from build123d import *

# Parameters (mm, degrees)
SKETCH1_W           = 96
SKETCH1_H           = 48
SKETCH1_R           = 2.05
BOSS_EXTRUDE1_DEPTH = 3.175
FILLET1_R           = 2


with BuildPart() as part:
    # Sketch1 → Boss-Extrude1 (new body)
    with BuildSketch(Plane.XY):
        Rectangle(SKETCH1_W, SKETCH1_H)
        with Locations((-40, 16)):
            Circle(SKETCH1_R, mode=Mode.SUBTRACT)
        with Locations((-8, 16)):
            Circle(SKETCH1_R, mode=Mode.SUBTRACT)
        with Locations((-8, -16)):
            Circle(SKETCH1_R, mode=Mode.SUBTRACT)
        with Locations((-40, -16)):
            Circle(SKETCH1_R, mode=Mode.SUBTRACT)
        with Locations((8, 16)):
            Circle(SKETCH1_R, mode=Mode.SUBTRACT)
        with Locations((8, -16)):
            Circle(SKETCH1_R, mode=Mode.SUBTRACT)
        with Locations((40, -16)):
            Circle(SKETCH1_R, mode=Mode.SUBTRACT)
        with Locations((40, 16)):
            Circle(SKETCH1_R, mode=Mode.SUBTRACT)
        with Locations((-36.7, 0)):
            Circle(SKETCH1_R, mode=Mode.SUBTRACT)
        with Locations((11.3, 0)):
            Circle(SKETCH1_R, mode=Mode.SUBTRACT)
        Polygon((-38.544929421, 20.05), (-30, 13), (-30, -13), (-38.544929421, -20.05), (-9.455070579, -20.05), (-18, -13), (-18, 13), (-9.455070579, 20.05), align=None, mode=Mode.SUBTRACT)
        Polygon((-11, -6), (-11, 6), (-4, 14.484327085), (4, 14.484327085), (4, -14.484327085), (-4, -14.484327085), align=None, mode=Mode.SUBTRACT)
        Polygon((38.544929421, -20.05), (30, -13), (30, 13), (38.544929421, 20.05), (9.455070579, 20.05), (18, 13), (18, -13), (9.455070579, -20.05), align=None, mode=Mode.SUBTRACT)
        Polygon((37, -6), (37, 6), (44, 14.484327085), (44, -14.484327085), align=None, mode=Mode.SUBTRACT)
    extrude(amount=BOSS_EXTRUDE1_DEPTH)

    # Fillet1
    fillet1_edges = [part.edges().sort_by_distance(p)[0] for p in [
        (-9.455070579, 20.05, 1.5875),
        (-38.544929421, 20.05, 1.5875),
        (-30, 13, 1.5875),
        (-30, -13, 1.5875),
        (-38.544929421, -20.05, 1.5875),
        (-9.455070579, -20.05, 1.5875),
        (-18, -13, 1.5875),
        (-18, 13, 1.5875),
        (38.544929421, 20.05, 1.5875),
        (9.455070579, 20.05, 1.5875),
        (18, 13, 1.5875),
        (18, -13, 1.5875),
        (9.455070579, -20.05, 1.5875),
        (38.544929421, -20.05, 1.5875),
        (30, -13, 1.5875),
        (30, 13, 1.5875),
        (-4, 14.484327085, 1.5875),
        (-11, 6, 1.5875),
        (-11, -6, 1.5875),
        (-4, -14.484327085, 1.5875),
        (4, -14.484327085, 1.5875),
        (4, 14.484327085, 1.5875),
        (37, -6, 1.5875),
        (44, -14.484327085, 1.5875),
        (44, 14.484327085, 1.5875),
        (37, 6, 1.5875),
        (-48, 24, 1.5875),
        (48, 24, 1.5875),
        (48, -24, 1.5875),
        (-48, -24, 1.5875),
    ]]
    fillet(fillet1_edges, radius=FILLET1_R)


solid = part.part
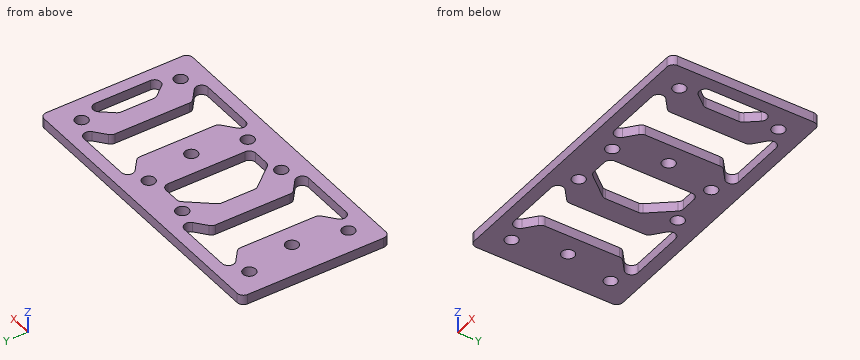
The model under review builds one solid part; all positions refer to its coordinate system, in mm. Coordinates: 2 decimals unless noted, no trailing zeros. Loops run counter-clockwise (first coordinate to the right, second up) from the corner with the lowest first, then second, coordinate; pieces in that order, holes last. Notation, with made-up numbers: M 10,45 L 34,45 A16 cw 34,64 Z; hole C 76.5,13.5 d4. An arc over 180 degrees is marked long. Put each result on its own line as item: value. Start each with the question number.
Q1. Add section C-C (x = -40). Write out the cut boundary in (y, z) (3 decimals), and give its area (3 significant figures).
Q2. Clearance check with a flat-ended pin moving along its axis: pin 1 (3.5 mm diameter, centred on x = -40, y = -16, fed in from +Z). State where the tip first meets the part, or that it passes through.
Q3. Add section B-B (y = 0). Write out the cut boundary in (x, z) (3 decimals).
Q4. Wall thickness on line 1 (X direction, y = -5, z = 1.2); line 2 (Y direction, x = 8, z = 1.05); line 3 (Y direction, x = 26, z = 1.4): over which ranges is each line inside the solid? List them lowest first.
Q5. Add section D-D (z = 2). Count the separate pieces of the cut face and the enclosed holes in it, and give its area (3 significant figures).
Q6. Add section A-A (x = 24). Write out the cut boundary in (y, z) (3 decimals), and give its area (3 significant figures).
Answers:
1. outline: M -24,0 L -18.05,0 L -18.05,3.175 L -24,3.175 Z; M -13.95,0 L 13.95,0 L 13.95,3.175 L -13.95,3.175 Z; M 18.05,0 L 24,0 L 24,3.175 L 18.05,3.175 Z
1. area: 126 mm^2
2. pin 1: passes through
3. outline: M -48,0 L -38.75,0 L -38.75,3.175 L -48,3.175 Z; M -34.65,0 L -30,0 L -30,3.175 L -34.65,3.175 Z; M -18,0 L -11,0 L -11,3.175 L -18,3.175 Z; M 4,0 L 9.25,0 L 9.25,3.175 L 4,3.175 Z; M 13.35,0 L 18,0 L 18,3.175 L 13.35,3.175 Z; M 30,0 L 37,0 L 37,3.175 L 30,3.175 Z; M 44,0 L 48,0 L 48,3.175 L 44,3.175 Z
4. line 1: x = -48 to -30, -18 to -11, 4 to 18, 30 to 37, 44 to 48
4. line 2: y = -24 to -18.05, -13.95 to 13.95, 18.05 to 24
4. line 3: y = -24 to -20.05, 20.05 to 24
5. separate pieces: 1
5. enclosed holes: 14
5. area: 2,810 mm^2
6. outline: M -24,0 L -20.05,0 L -20.05,3.175 L -24,3.175 Z; M 20.05,0 L 24,0 L 24,3.175 L 20.05,3.175 Z
6. area: 25.1 mm^2
